Here's how the part is built. I have some questions about the finished solid (model axes, mm). Give positions to 0.01 mm unless a question says otherwise; leave off trailing zeros. Write each loop counter-clockwise with the first axis right and the second up, starting at its lowest first coordinate (ties: lowest second). Pieces come first, ordered by that corner, then holes. Notation, with made-up numbers: (-21.5, 88.5) - (-13.5, 88.5) arc R11 ccw to (-13.5, 92.5) - close; hole circle Ø11 at (38, 41). An arc over 180 degrees is marked (long way). One line per item, written item: value. Start each with the question number.
1) Imagine slicing it at A-A on x = 106.5. Write out the boundary of the cut face in (y, z), plus the area to 3 significant figures.
2) Please list where these lines run through material, in increasing order: L1, parallel to X at y = 894, z = 4.25; L2, parallel to Y at x = 106.5, z = 3.5; L3, parallel to Y at x = -71.5, z = 3.5. Write a range as [from, to].
3) Imagine slicing it at D-D on x = 760. Write out the boundary of the cut face in (y, z).
4) Imagine slicing it at C-C on y = 1790. Write out the boundary of the cut face in (x, z).
5) I'm going to push flat-ended pins straight in: P1, Ø11.5, axis at x = -51.7, y = 1209.91, coming from the -Z side; P2, Ø1.5, axis at y = 1613, z = 8.5, coming from the +X side; P3, Ø1, axis at y = 1470.5, z = 6, coming from the +X side. Where does each tip first touch, or does it pass through?
Autodesk Inventor part; units mm, degrees
ref_plane "YZ Plane" through (0, 0, 0) normal (1, 0, 0) x (0, 1, 0)
ref_plane "XZ Plane" through (0, 0, 0) normal (0, 1, 0) x (-1, 0, 0)
ref_plane "XY Plane" through (0, 0, 0) normal (0, 0, 1) x (1, 0, 0)
sketch "Sketch1" plane through (0, 0, 0) normal (0, 0, 1) x (1, 0, 0)
  line L0 (0, 0) -> (0, 1910) construction
  line L1 (424.5155, 1910) -> (-415.4845, 1910)
  line L2 (-415.4845, 1910) -> (-1180, 1150)
  line L3 (-1180, 0) -> (-1180, 1150)
  line L4 (960, 0) -> (960, 1342.8524)
  line L5 (424.5155, 1910) -> (960, 1342.8524)
  circle A0 centre (0, 950) radius 265 construction
  line L6 (960, 0) -> (-1180, 0)
  circle A1 centre (-1701.6377, -269.2167) radius 188.5 construction
  circle A2 centre (-800, 80) radius 55
  circle A3 centre (0, 950) radius 170
  line L7 (0, 1215) -> (0, 1120) construction
  line L8 (-721.2646, 955) -> (721.2646, 955) construction
  line L9 (-169.9265, 955) -> (-174.9265, 955) construction
  line L10 (-174.9265, 960) -> (-174.9265, 950)
  line L11 (-174.9265, 960) -> (-169.7056, 960)
  line L12 (-174.9265, 950) -> (-170, 950)
  line L13 (169.9265, 955) -> (174.9265, 955) construction
  line L14 (174.9265, 960) -> (174.9265, 950)
  line L15 (169.7056, 960) -> (174.9265, 960)
  line L16 (174.9265, 950) -> (170, 950)
  line L17 (-174.9265, 970) -> (174.9265, 970)
  line L18 (174.9265, 970) -> (174.9265, 940)
  line L19 (174.9265, 940) -> (-174.9265, 940)
  line L20 (-174.9265, 940) -> (-174.9265, 970)
  arc A4 (-2.4999, 780.0184) -> (2.4999, 780.0184) centre (0, 780) ccw
  arc A5 (2.4999, 1119.9816) -> (-2.4999, 1119.9816) centre (0, 1120) ccw
  point P0 (0, 955)
  point P1 (-169.7056, 940)
  point P2 (169.7056, 940)
  point P3 (168.8194, 970)
  point P4 (-168.8194, 970)
  dimension "d52" = 530
  dimension "d72" = 340
  dimension "d1" = 840
  dimension "d3" = 1150
  dimension "d12" = 1180
  dimension "d13" = 950
  dimension "d14" = 110
  dimension "d15" = 1910
  dimension "d17" = -521.6377
  dimension "d18" = 377
  dimension "d19" = -269.2167
  dimension "d34" = 380
  dimension "d35" = 80
  dimension "d37" = 2140
  dimension "d53" = 5
  dimension "d54" = 10
  dimension "d55" = 30
  dimension "d67" = 5
  dimension "d68" = 5
  dimension "d69" = 780
  dimension "d71" = 1078
extrude "Extrusion1" add sketch "Sketch1" along normal blind 10 contours L5 L4 L6 L3 L2 L1 | A3 L19 L17 | L16 L18 L19 A3 | A3 L15 L14 L16 | A3 L17 L18 L15 | L19 L20 L12 A3 | A3 L11 L20 L17 | L12 L10 L11 A3
fillet "Fillet1" radius 10 4 edges at (-168.8194, 970, 5) (-169.7056, 940, 5) (168.8194, 970, 5) (169.7056, 940, 5)
sketch "Sketch4" plane through (0, 0, 0) normal (0, 0, 1) x (1, 0, 0)
  circle A0 centre (-51.6989, 1209.9081) radius 6.5
  arc A1 (-2.4999, 1119.9816) -> (-166.985, 981.875) centre (0, 950) ccw
  line L0 (0, 950) -> (0, 1196.7062) construction
  line L1 (-51.6989, 1209.9081) -> (0, 950) construction
  point P0 (0, 0)
  point P1 (-5, 1149.9375)
  dimension "d59" = 265
  dimension "d60" = 13
  dimension "d61" = 11.25
extrude "Extrusion4" cut sketch "Sketch4" along normal blind 10
pattern_circular "Circular Pattern3" count 16 over 360 about axis through (0, 950, 0) along (0, 0, 1) of "Extrusion4"
sketch "Sketch5" plane through (0, 0, 10) normal (0, 0, 1) x (1, 0, 0)
  circle A0 centre (51.6989, 1209.9081) radius 6.5
  circle A1 centre (147.2261, 1170.3394) radius 6.5
  circle A2 centre (220.3394, 1097.2261) radius 6.5
  circle A3 centre (259.9081, 1001.6989) radius 6.5
  circle A4 centre (259.9081, 898.3011) radius 6.5
  circle A5 centre (220.3394, 802.7739) radius 6.5
  circle A6 centre (147.2261, 729.6606) radius 6.5
  circle A7 centre (51.6989, 690.0919) radius 6.5
  circle A8 centre (-51.6989, 690.0919) radius 6.5
  circle A9 centre (-147.2261, 729.6606) radius 6.5
  circle A10 centre (-220.3394, 802.7739) radius 6.5
  circle A11 centre (-259.9081, 898.3011) radius 6.5
  circle A12 centre (-259.9081, 1001.6989) radius 6.5
  circle A13 centre (-220.3394, 1097.2261) radius 6.5
  circle A14 centre (-147.2261, 1170.3394) radius 6.5
  circle A15 centre (-51.6989, 1209.9081) radius 6.5
  line L0 (960, 1342.8524) -> (424.5155, 1910)
  line L1 (424.5155, 1910) -> (-415.4845, 1910)
  line L2 (-415.4845, 1910) -> (-1180, 1150)
  line L3 (-1180, 1150) -> (-1180, 0)
  line L4 (-1180, 0) -> (960, 0)
  line L5 (960, 0) -> (960, 1342.8524)
  arc A16 (2.4999, 780.0184) -> (168.6666, 928.75) centre (0, 950) ccw
  arc A17 (-2.4999, 780.0184) -> (2.4999, 780.0184) centre (0, 780) ccw
  arc A18 (-168.6666, 928.75) -> (-2.4999, 780.0184) centre (0, 950) ccw
  arc A19 (-158.7451, 940) -> (-168.6666, 928.75) centre (-158.7451, 930) ccw
  line L6 (-158.7451, 940) -> (158.7451, 940)
  arc A20 (168.6666, 928.75) -> (158.7451, 940) centre (158.7451, 930) ccw
  circle A21 centre (-800, 80) radius 55
  line L7 (157.1623, 970) -> (-157.1623, 970)
  arc A22 (-166.985, 981.875) -> (-157.1623, 970) centre (-157.1623, 980) ccw
  arc A23 (-2.4999, 1119.9816) -> (-166.985, 981.875) centre (0, 950) ccw
  arc A24 (2.4999, 1119.9816) -> (-2.4999, 1119.9816) centre (0, 1120) ccw
  arc A25 (166.985, 981.875) -> (2.4999, 1119.9816) centre (0, 950) ccw
  arc A26 (157.1623, 970) -> (166.985, 981.875) centre (157.1623, 980) ccw
  line L8 (-380, 0) -> (-380, 1910)
  point P0 (0, 0)
  dimension "d73" = 1340
extrude "Extrusion5" cut sketch "Sketch5" against normal through all contours L8 L4 L3 L2 L1
properties part number "ДМФ 012 Стенка Корма ПРАВ v2.0"
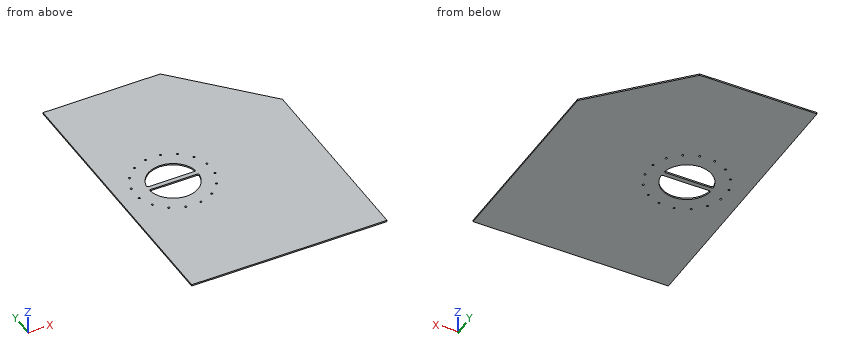
Numbers:
1. outline: (0, 0) - (817.49, 0) - (817.49, 10) - (0, 10) - close; (940, 0) - (970, 0) - (970, 10) - (940, 10) - close; (1082.51, 0) - (1910, 0) - (1910, 10) - (1082.51, 10) - close
1. area: 16,700 mm^2
2. L1: [-380, -264.78], [-255.03, -160.51], [160.51, 255.03], [264.78, 960]
2. L2: [0, 817.49], [940, 970], [1082.51, 1910]
2. L3: [0, 795.77], [940, 970], [1104.23, 1910]
3. outline: (0, 0) - (1554.68, 0) - (1554.68, 10) - (0, 10) - close
4. outline: (-380, 0) - (537.82, 0) - (537.82, 10) - (-380, 10) - close
5. P1: through
5. P2: x = 705.64
5. P3: x = 839.95
